from build123d import *

# Parameters (mm, degrees)
EXTRUDE_1_DEPTH     = 66
HOLE_WIZARD_1_D     = 5.2
HOLE_WIZARD_1_DEPTH = 100


with BuildPart() as part:
    # 草图1 → 凸台-拉伸1 (new body)
    with BuildSketch(Plane.XY):
        Polygon((-15, -1.5), (-13.1, -1.5), (-13.1, -21.5), (-10.1, -21.5), (-10.1, -1.5), (10.1, -1.5), (10.1, -21.5), (13.1, -21.5), (13.1, -1.5), (15, -1.5), (15, 1.5), (-15, 1.5), align=None)
    extrude(amount=EXTRUDE_1_DEPTH)

    # 孔1
    with Locations(Plane(origin=(13.1, 0, 0), x_dir=(0, 0, -1), z_dir=(1, 0, 0))):
        with Locations((-50, -11.5), (-30, -11.5), (-12, -11.5)):
            Hole(HOLE_WIZARD_1_D / 2, depth=HOLE_WIZARD_1_DEPTH)


solid = part.part
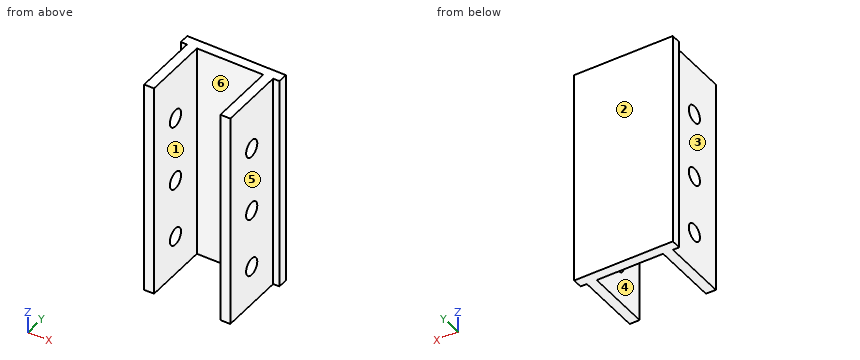
The listing builds one solid part. Answer for the finished solid, in the listing's coordinates (mm). Face numbers are marked on the shaded views. A direction names the side the tool comes from. Coordinates: 2 decimals unless noted, no trailing zeros. Loops run counter-clockwise (first coordinate to the right, second up) from the corner with the lowest first, then second, coordinate; pieces in that order, holes last.
1) Find section B-B on z = 12. Write down the section's boundary in (x, y).
2) Find section A-A on y = -10.5. Give the number of separate pieces and of enclosed holes in the cut face, then the cut area to 3 significant figures.
3) Flat-ended cylindrical pins translate along their axes: pin 1 Ø1.5 at (x, z) = (14, 32) entering from -Y; pin 2 Ø6 at (y, z) = (-9.5, 25) entering from -X; pin 3 Ø7 at (y, z) = (-11.5, 50) entering from +X. Find the tip coordinate at first contact, or state that the pin passes through.
4) Determine the mould class of the marked faces 3, 4, 5 and 6 for opening direction X: pulls with the +X half, pulls with the -X half, needs draft (parallel to the pull), parting line crosses it, or undercut.
5) Find section C-C on y = -17.75. Write down the section's boundary in (x, z).
6) Find section D-D on z = 4. Write down the section's boundary in (x, y), then the cut area to 3 significant figures.
7) Find the intervals of material crossed by L1, parallel to X at y = -4, z = 14; L2, parallel to Y at x = -11.8, z = 50; L3, parallel to Y at x = 1.5, z = 33, in increasing order.
8) A tool of negligible diameter and unlimited length cuts with its end or side. For the marked faces 1 and 2, from which of +Z, -Z, +X, -X, +Y, -Y can it reach the whole face along a straight path? Write none if from no direction.
Values:
1. outline: (-15, -1.5) - (-13.1, -1.5) - (-13.1, -8.9) - (-10.1, -8.9) - (-10.1, -1.5) - (10.1, -1.5) - (10.1, -8.9) - (13.1, -8.9) - (13.1, -1.5) - (15, -1.5) - (15, 1.5) - (-15, 1.5) - close; (-13.1, -21.5) - (-10.1, -21.5) - (-10.1, -14.1) - (-13.1, -14.1) - close; (10.1, -21.5) - (13.1, -21.5) - (13.1, -14.1) - (10.1, -14.1) - close
2. separate pieces: 8
2. enclosed holes: 0
2. area: 310 mm2
3. pin 1: stops at y = -1.5
3. pin 2: stops at x = -13.1
3. pin 3: stops at x = 13.1
4. face 3: pulls with the -X half
4. face 4: undercut
4. face 5: pulls with the +X half
4. face 6: undercut
5. outline: (-13.1, 0) - (-10.1, 0) - (-10.1, 66) - (-13.1, 66) - close; (10.1, 0) - (13.1, 0) - (13.1, 66) - (10.1, 66) - close
6. outline: (-15, -1.5) - (-13.1, -1.5) - (-13.1, -21.5) - (-10.1, -21.5) - (-10.1, -1.5) - (10.1, -1.5) - (10.1, -21.5) - (13.1, -21.5) - (13.1, -1.5) - (15, -1.5) - (15, 1.5) - (-15, 1.5) - close
6. area: 210 mm2
7. L1: x = -13.1 to -10.1, 10.1 to 13.1
7. L2: y = -21.5 to -14.1, -8.9 to 1.5
7. L3: y = -1.5 to 1.5
8. face 1: +Z, -Z, -Y
8. face 2: +Z, -Z, +X, -X, +Y
